Check sheet for the modelled part. Datum: model origin and axes. Units: mm. Face numbers are marked on the shaded views. A direction names the side the tool comes from. Round coordinates to 2 decimals unless told otherwise and drop trailing zeros. Loops run counter-clockwise (first coordinate to the right, second up) from the corner with the lowest first, then second, coordinate; pieces in that order, holes last. Notation, with made-up numbers: (-2.5, 41.25) - (9.5, 41.25) arc R7 cw to (9.5, 46.25) - close; hole circle Ø5 at (34.5, 79.5). An arc over 180 degrees is marked (long way). Answer in a Markdown table with one row per item. Add a question column.
(1) Access from +Z, -Z, +X, -X, +Y, -Y to the whole of each face (thin tool, end or side, straight path). Record for the marked faces 1 and 2.
(2) Thickness scan on line 1 along X through (y, z) = (18, 20.5); line 2 along Z through (x, y) = (0, -1); line 3 along Z through (x, y) = (-26.55, 12.5). Record the ranges inside material, lowest first.
(3) Cross-section at D-D on y = 14. Enter the section's corners in (x, z), then the cut area to 3 significant figures.
(4) Cross-section at B-B on y = 6. Enter the section's corners in (x, z).
(5) Cross-section at C-C on z = 12.75. Enter the section's corners in (x, y), then the cut area to 3 significant figures.
(6) Mould release check, pull along X, two halves, no side actions. Record for the marked faces 3, 4, 5 and 6: +X half, -X half, draft (parallel to the pull), parting line (faces both ways), or undercut.
(7) Cross-section at A-A on x = 0. Enter the section's corners in (y, z), then the cut area to 3 significant figures.
(8) Gauge pin test, flat ends, axial feed: pin 1 (4.5 mm diameter, centred on y = 25, z = 8, fed in from -X); pin 2 (20.5 mm diameter, centred on x = -7.5, z = 16, fed in from +Y). Record the tip position at first contact, or that the pin passes through.
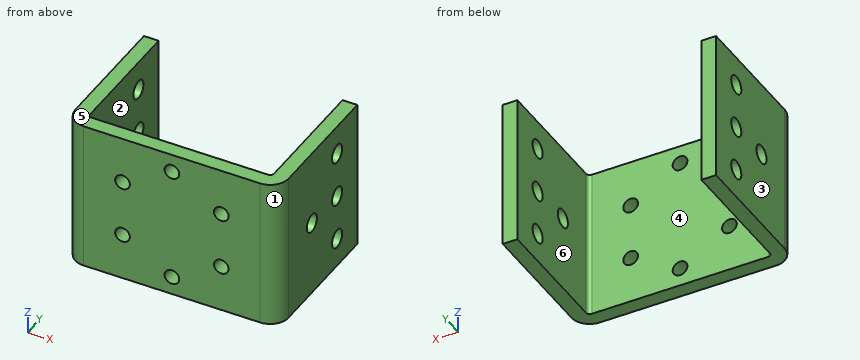
from build123d import *

# Parameters (mm, degrees)
SM_BASE_FLANGE_1_DEPTH   = 41
SKETCH_9_R               = 2
CUT_EXTRUDE_4_DEPTH      = 64.584589328
CUT_EXTRUDE_5_DEPTH      = 80.183331579
CUT_EXTRUDE_5_DEPTH_BACK = 80.183331579
SKETCH_10_R              = 2.5


# Sheet-metal steps are written as plain solids
with BuildPart() as part:
    # Sketch 1 → Базовая кромка1 (new body)
    with BuildSketch(Plane.XY):
        with BuildLine():
            Line((-25, 35), (-25, 1))
            ThreePointArc((-25, 1), (-24.707106781, 0.292893219), (-24, 0))
            Line((-24, 0), (24, 0))
            ThreePointArc((24, 0), (24.707106781, 0.292893219), (25, 1))
            Line((25, 1), (25, 35))
            Line((25, 35), (29, 35))
            Line((29, 35), (29, 1))
            ThreePointArc((29, 1), (27.535533906, -2.535533906), (24, -4))
            Line((24, -4), (-24, -4))
            ThreePointArc((-24, -4), (-27.535533906, -2.535533906), (-29, 1))
            Line((-29, 1), (-29, 35))
            Line((-29, 35), (-25, 35))
        make_face()
    extrude(amount=SM_BASE_FLANGE_1_DEPTH)

    # Эскиз9 → Вырез-Вытянуть4 (cut, through all)
    with BuildSketch(Plane.XZ.offset(4)):
        with Locations((0, 5)):
            Circle(SKETCH_9_R)
        with Locations((-13.423393759, 12.75)):
            Circle(SKETCH_9_R)
        with Locations((-13.423393759, 28.25)):
            Circle(SKETCH_9_R)
        with Locations((0, 36)):
            Circle(SKETCH_9_R)
        with Locations((13.423393759, 28.25)):
            Circle(SKETCH_9_R)
        with Locations((13.423393759, 12.75)):
            Circle(SKETCH_9_R)
    extrude(amount=-CUT_EXTRUDE_4_DEPTH, mode=Mode.SUBTRACT)

    # Эскиз10 → Вырез-Вытянуть5 (cut, two sides: drawn at the far end of the back side and taken through both)
    with BuildSketch(Plane(origin=(29, 0, 0), x_dir=(0, 0, -1), z_dir=(1, 0, 0)).offset(-CUT_EXTRUDE_5_DEPTH_BACK)):
        with Locations((-33, 25)):
            Circle(SKETCH_10_R)
        with Locations((-20.5, 25)):
            Circle(SKETCH_10_R)
        with Locations((-8, 25)):
            Circle(SKETCH_10_R)
        with Locations((-20.5, 12.5)):
            Circle(SKETCH_10_R)
    extrude(amount=CUT_EXTRUDE_5_DEPTH + CUT_EXTRUDE_5_DEPTH_BACK, mode=Mode.SUBTRACT)


solid = part.part
Answers:
| question | item | result |
|---|---|---|
| 1 | face 1 | +Z, -Z, +X, -Y |
| 1 | face 2 | +Z, -Z, +Y |
| 2 | line 1 | x = -29 to -25, 25 to 29 |
| 2 | line 2 | z = 0 to 3, 7 to 34, 38 to 41 |
| 2 | line 3 | z = 0 to 18, 23 to 41 |
| 3 | outline | (-29, 0) - (-25, 0) - (-25, 18.5) - (-29, 18.5) - close; (-29, 22.5) - (-25, 22.5) - (-25, 41) - (-29, 41) - close; (25, 0) - (29, 0) - (29, 18.5) - (25, 18.5) - close; (25, 22.5) - (29, 22.5) - (29, 41) - (25, 41) - close |
| 3 | area | 296 mm^2 |
| 4 | outline | (-29, 0) - (-25, 0) - (-25, 41) - (-29, 41) - close; (25, 0) - (29, 0) - (29, 41) - (25, 41) - close |
| 5 | outline | (-29, 1) arc R5 ccw to (-24, -4) - (-15.42, -4) - (-15.42, 0) - (-24, 0) arc R1 cw to (-25, 1) - (-25, 35) - (-29, 35) - close; (-11.42, -4) - (11.42, -4) - (11.42, 0) - (-11.42, 0) - close; (15.42, -4) - (24, -4) arc R5 ccw to (29, 1) - (29, 35) - (25, 35) - (25, 1) arc R1 cw to (24, 0) - (15.42, 0) - close |
| 5 | area | 470 mm^2 |
| 6 | face 3 | -X half |
| 6 | face 4 | undercut |
| 6 | face 5 | draft |
| 6 | face 6 | undercut |
| 7 | outline | (-4, 0) - (0, 0) - (0, 3) - (-4, 3) - close; (-4, 7) - (0, 7) - (0, 34) - (-4, 34) - close; (-4, 38) - (0, 38) - (0, 41) - (-4, 41) - close |
| 7 | area | 132 mm^2 |
| 8 | pin 1 | passes through |
| 8 | pin 2 | stops at y = 0 |
